Here's how the part is built. I have some questions about the finished solid (model axes, mm). A direction names the side the tool comes from. Coordinates: 2 decimals unless noted, no trailing zeros. Write each loop counter-clockwise with the first axis right and the second up, starting at its lowest first coordinate (ties: lowest second). Pieces come first, ordered by that corner, then holes.
Item 1: If we section it at A-A (z = 7.5): Please give me the cut outline in (x, y) (1 decimal).
Item 2: If I drill on line 1 (Y direction, x = -3.25, z = 8.25); line 2 (X direction, y = -22, z = 9.5); line 3 (Y direction, x = -2, z = 7.75), over which ranges is the centre line in solid material (lowest first)?
Item 3: If we section it at C-C (y = -26): Please give me the cut outline in (x, z).
Item 4: For faces 1 (the face through (-1, -5, 10)), 2 (the face through (-7, -14, 20)), 3 (the face through (-7, -24, 10)), which set-ups out of +Z, -Z, +X, -X, +Y, -Y let a thin tool reach every point of the face, with its end or its side?
Item 5: If we section it at D-D (z = 1.5): Please give me the cut outline in (x, y) (1 decimal).
Item 6: If we section it at B-B (x = -4.5): Please give me the cut outline in (y, z).
Item 7: I'm going to push flat-ended pins straight in: pin 1 Ø11 at (y, z) = (-7, 6) entering from -X; pin 2 Ø12 at (y, z) = (-25.5, 16) entering from +X; pin 3 Ø2.5 at (x, z) = (-5, 12) entering from +Y. Where does each tip first touch, or does it pass through?
from build123d import *

# Parameters (mm, degrees)
BOSS_EXTRUDE1_DEPTH = 20
CUT_EXTRUDE1_DEPTH  = 55


with BuildPart() as part:
    # Sketch1 → Boss-Extrude1 (new body)
    with BuildSketch(Plane.XY):
        with BuildLine():
            Line((-1, 0), (-1, -10.1125))
            ThreePointArc((-1, -10.1125), (-1.464967985, -11.235032015), (-2.5875, -11.7))
            Line((-2.5875, -11.7), (-7.4125, -11.7))
            ThreePointArc((-7.4125, -11.7), (-8.535032015, -12.164967985), (-9, -13.2875))
            Line((-9, -13.2875), (-9, -32.7))
            ThreePointArc((-9, -32.7), (-8, -33.7), (-7, -32.7))
            Line((-7, -32.7), (-7, -15.2875))
            ThreePointArc((-7, -15.2875), (-6.535032015, -14.164967985), (-5.4125, -13.7))
            Line((-5.4125, -13.7), (-0.5875, -13.7))
            ThreePointArc((-0.5875, -13.7), (0.535032015, -13.235032015), (1, -12.1125))
            Line((1, -12.1125), (1, 0))
            ThreePointArc((1, 0), (0, 1), (-1, 0))
        make_face()
    extrude(amount=BOSS_EXTRUDE1_DEPTH)

    # Sketch2 → Cut-Extrude1 (cut)
    with BuildSketch(Plane.ZY.offset(9)):
        with BuildLine():
            ThreePointArc((0, -5.35), (1.859871939, -0.859871939), (6.35, 1))
            Line((6.35, 1), (0, 1))
            Line((0, 1), (0, -5.35))
        make_face()
        with BuildLine():
            Line((20, 1), (13.65, 1))
            ThreePointArc((13.65, 1), (18.140128061, -0.859871939), (20, -5.35))
            Line((20, -5.35), (20, 1))
        make_face()
        with BuildLine():
            Line((20, -32.7), (20, -27.35))
            ThreePointArc((20, -27.35), (19.219687686, -30.399767053), (17.070526275, -32.7))
            Line((17.070526275, -32.7), (20, -32.7))
        make_face()
        with BuildLine():
            Line((20, -33.7), (20, -32.7))
            Line((20, -32.7), (17.070526275, -32.7))
            ThreePointArc((17.070526275, -32.7), (15.431852968, -33.444874896), (13.65, -33.7))
            Line((13.65, -33.7), (20, -33.7))
        make_face()
        with BuildLine():
            ThreePointArc((2.929473725, -32.7), (0.780312314, -30.399767053), (0, -27.35))
            Line((0, -27.35), (0, -32.7))
            Line((0, -32.7), (2.929473725, -32.7))
        make_face()
        with BuildLine():
            Line((2.929473725, -32.7), (0, -32.7))
            Line((0, -32.7), (0, -33.7))
            Line((0, -33.7), (6.35, -33.7))
            ThreePointArc((6.35, -33.7), (4.568147032, -33.444874896), (2.929473725, -32.7))
        make_face()
    extrude(amount=-CUT_EXTRUDE1_DEPTH, mode=Mode.SUBTRACT)


solid = part.part
Answer list:
1. outline: (-9, -32.7) arc R1 ccw to (-7, -32.7) - (-7, -15.3) arc R1.6 cw to (-5.4, -13.7) - (-0.6, -13.7) arc R1.6 ccw to (1, -12.1) - (1, 0) arc R1 ccw to (-1, 0) - (-1, -10.1) arc R1.6 cw to (-2.6, -11.7) - (-7.4, -11.7) arc R1.6 ccw to (-9, -13.3) - close
2. line 1: y = -13.7 to -11.7
2. line 2: x = -9 to -7
2. line 3: y = -13.7 to -11.59
3. outline: (-9, 0) - (-7, 0) - (-7, 20) - (-9, 20) - close
4. face 1: +Z, -Z, -X, +Y
4. face 2: +Z, +X, -X, +Y, -Y
4. face 3: +Z, -Z, +X, -Y
5. outline: (-9, -31.4) - (-7, -31.4) - (-7, -15.3) arc R1.6 cw to (-5.4, -13.7) - (-0.6, -13.7) arc R1.6 ccw to (1, -12.1) - (1, -1.3) - (-1, -1.3) - (-1, -10.1) arc R1.6 cw to (-2.6, -11.7) - (-7.4, -11.7) arc R1.6 ccw to (-9, -13.3) - close
6. outline: (-13.7, 0) - (-11.7, 0) - (-11.7, 20) - (-13.7, 20) - close
7. pin 1: stops at x = -8.79
7. pin 2: stops at x = -7
7. pin 3: stops at y = -11.7
